Geometry: see drawing. Coordinates: mm, zero at the bounding-box minimum. A direction names the side the tool comes from. Coordinates: 2 decimals unless noted, no trailing zeros. Write each loop counter-clockwise with the first axis right and the second up, starting at its lowest first coordinate (ties: lowest second). Pieces come first, ordered by that corner, then holes. Notation, with made-up numbers: (75, 46.5) -> (134, 46.5) arc R23 cw to (134, 68.5) -> close; hole circle Ø4 at (77, 5). An arc over 180 degrees is marked (long way). Answer as a JSON object with one key per item and string values. Group by question number.
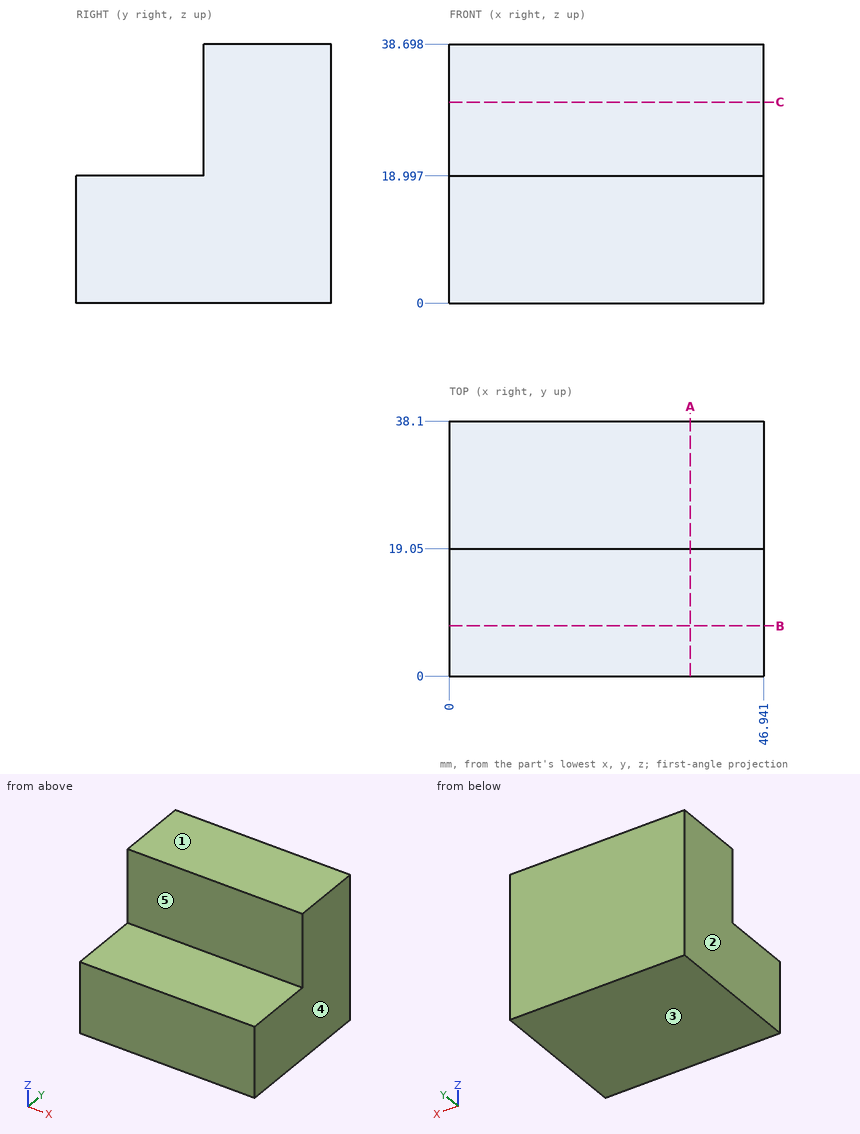
Item 1: Contact query for flat-ended pins moving along their axis: pin 1 (12 mm diameter, centred on x = 37, y = 16.5, fed in from +Z); pin 2 (15 mm diameter, centred on x = 23.5, y = 7.5, fed in from +Z); pin 3 (1 mm diameter, centred on x = 26, z = 32.5, fed in from -Y). Output: stop coordinate, or through.
Item 2: Section C-C on z = 30. Output: boundary loops of the cut face in (x, y), then the cut area to 3 significant figures.
Item 3: Section A-A on x = 36. Output: boundary loops of the cut face in (y, z).
Item 4: Section B-B on y = 7.5. Output: boundary loops of the cut face in (x, z), then the cut area to 3 significant figures.
Item 5: Set-up query: the marked faces 4 and 5. Return all of +Z, -Z, +X, -X, +Y, -Y with unobstructed straight access to the full face (end or side cutting, diameter ignored); none if empty.
Item 6: Mould query, pull axis Z, two halves, no side actions, for the marked faces 1, 2 and 3. Classes: +Z half, -Z half, draft (parallel to the pull), parting line (faces both ways), or undercut.
Item 7: Ray query, L1, parallel to Y at x = 37, z = 28; L2, parallel to Z at x = 43.5, y = 8.5. Return the intervals inside material, ascending. Write a range as [from, to].
Answer sheet:
{
 "1": {"pin 1": "stops at z = 38.7", "pin 2": "stops at z = 19", "pin 3": "stops at y = 19.05"},
 "2": {"outline": "(0, 19.05) -> (46.94, 19.05) -> (46.94, 38.1) -> (0, 38.1) -> close", "area": "894 mm^2"},
 "3": {"outline": "(0, 0) -> (38.1, 0) -> (38.1, 38.7) -> (19.05, 38.7) -> (19.05, 19) -> (0, 19) -> close"},
 "4": {"outline": "(0, 0) -> (46.94, 0) -> (46.94, 19) -> (0, 19) -> close", "area": "892 mm^2"},
 "5": {"face 4": "+Z, -Z, +X, +Y, -Y", "face 5": "+Z, +X, -X, -Y"},
 "6": {"face 1": "+Z half", "face 2": "draft", "face 3": "-Z half"},
 "7": {"L1": "y = [19.05, 38.1]", "L2": "z = [0, 19]"}
}
